from build123d import *

# Parameters (mm, degrees)
F0_W     = 25
F0_H     = 25
F1_DEPTH = 400
F2_W     = 21
F2_H     = 21
F3_DEPTH = 800.001
F4_W     = 21
F4_H     = 90
F5_DEPTH = 25.001
F7_DEPTH = 25.001


with BuildPart() as f1:
    # F0 (on Top) → F1 (new body, symmetric)
    with BuildSketch(Plane.XY):
        Rectangle(F0_W, F0_H)
    extrude(amount=F1_DEPTH, both=True)

    # F2 (on face) → F3 (cut, through all)
    with BuildSketch(Plane.XY.offset(400)):
        Rectangle(F2_W, F2_H)
    extrude(amount=-F3_DEPTH, mode=Mode.SUBTRACT)

    # F4 (on face) → F5 (cut, through all)
    with BuildSketch(Plane(origin=(-12.5, 0, 0), x_dir=(0, -1, 0), z_dir=(-1, 0, 0))):
        with Locations((0, 355)):
            Rectangle(F4_W, F4_H)
    extrude(amount=-F5_DEPTH, mode=Mode.SUBTRACT)

    # F6 (on face) → F7 (cut, through all)
    with BuildSketch(Plane.XZ.offset(12.5)):
        with BuildLine():
            Line((6, 380), (6, 400))
            Line((6, 400), (-6, 400))
            Line((-6, 400), (-6, 380))
            ThreePointArc((-6, 380), (0, 374), (6, 380))
        make_face()
    extrude(amount=-F7_DEPTH, mode=Mode.SUBTRACT)


solid = f1.part
Verification items for the finished model (mm, model axes). A direction names the side the tool comes from. Give positions to 0.01 mm unless a question says otherwise; leave off trailing zeros. Loops run counter-clockwise (first coordinate to the right, second up) from the corner with the lowest first, then second, coordinate; pieces in that order, holes last.
1) Depth check by flat-ended pin: pin 1 Ø1.6 at (x, y) = (11.5, -4.5) entering from +Z. Enter the tip coordinate at first touch or a pass-through.
2) Sectioned sample at B-B, the plane y = 5. Enter the section's corners in (x, z).
3) Set-up check for faces 1 (the flat face through (10.5, 0, -40)), 2 (the flat face through (0, -12.5, 6)): record each of +Z, -Z, +X, -X, +Y, -Y from which the full face is reachable in a straight line by a thin tool's end or side.
4) Sectioned sample at A-A, the plane x = 0. Enter the section's corners in (y, z).
5) Thickness scan on line 1 along Y through (x, z) = (2.75, 177.5); line 2 along Z through (x, y) = (-11, 7.5). Record the ranges inside material, lowest first.
6) Draft check along X on faces 3 (the flat face through (-12.5, 0, 6)), 4 (the flat face through (12.5, 0, 6)), 5 (the flat face through (0, 10.5, -6)). Enter one of: pulls with the +X half, pulls with the -X half, needs draft (parallel to the pull), parting line crosses it, or undercut.
7) Sectioned sample at C-C, the plane z = 281.5. Enter the section's corners in (x, y).
Answers:
1. pin 1: stops at z = 310
2. outline: (-12.5, -400) - (-10.5, -400) - (-10.5, 310) - (-12.5, 310) - close; (10.5, -400) - (12.5, -400) - (12.5, 310) - (10.5, 310) - close
3. face 1: +Z, -Z
3. face 2: +Z, -Z, +X, -X, -Y
4. outline: (-12.5, -400) - (-10.5, -400) - (-10.5, 374) - (-12.5, 374) - close; (10.5, -400) - (12.5, -400) - (12.5, 374) - (10.5, 374) - close
5. line 1: y = -12.5 to -10.5, 10.5 to 12.5
5. line 2: z = -400 to 310
6. face 3: pulls with the -X half
6. face 4: pulls with the +X half
6. face 5: undercut
7. outline: (-12.5, -12.5) - (12.5, -12.5) - (12.5, 12.5) - (-12.5, 12.5) - close; hole (-10.5, -10.5) - (10.5, -10.5) - (10.5, 10.5) - (-10.5, 10.5) - close
